For this review, take the finished solid that the model builds, in its own axes (mm). Coordinates: 2 decimals unless noted, no trailing zeros. Order: outer loops, then holes, each group sorted by start corner. A loop starts at its lowest first (then second) coordinate and runs counter-clockwise, first axis right, second up. Notation, with made-up numbers: (28.5, 20.25) -> (57.5, 20.25) arc R31 ccw to (57.5, 47.25) -> close; hole circle Ø11 at (24, -37). An arc over 180 degrees is marked (long way). Answer as a JSON object with one key per item and string values. Group by question number.
1) Draft analysis for pull direction Z (two halves, no side actions). For faces 1 (the flat face through (0, 6, 0)), 2 (the flat face through (0, 3, 2)), 3 (the cylindrical face through (-11.976, 5.423, 6.368)), state which applies: +Z half, -Z half, draft (parallel to the pull), parting line (faces both ways), or undercut.
2) For pin 1 (1.5 mm diameter, centred on x = -3.5, z = 3.5, fed in from -Y), flat-tipped, find the tip position at first contact; note if it passes through.
3) Add section A-A, the plane x = 0. Write out the cut boundary in (y, z), then the cut area to 3 significant figures.
4) Add section D-D, the plane x = -13.5. Write out the cut boundary in (y, z), then the cut area to 3 significant figures.
5) Wall thickness on L1, parallel to Z at x = 13.5, y = 5.75; L2, parallel to Z at x = -15, y = 9.5; L3, parallel to X at y = 8.25, z = 15.75: over which ranges is each line inside the solid? List them lowest first.
6) Add section B-B, the plane y = 9.75. Write out the cut boundary in (x, z), then the cut area to 3 significant figures.
7) Add section C-C, the plane z = 12. Write out the cut boundary in (x, y), then the cut area to 3 significant figures.
from build123d import *

# Parameters (mm, degrees)
EXTRUDE_1_DEPTH     = 22
SKETCH_3_R          = 1.65
CUT_EXTRUDE_2_DEPTH = 19
EXTRUDE_2_DEPTH     = 2
SKETCH_5_R          = 1.65
CUT_EXTRUDE_3_DEPTH = 31.186917806


with BuildPart() as part:
    # 草图1 → 凸台-拉伸1 (new body)
    with BuildSketch(Plane.XY):
        with BuildLine():
            Line((-10.583005244, 3), (-17.5, 3))
            Line((-17.5, 3), (-17.5, 0))
            Line((-17.5, 0), (-11, 0))
            ThreePointArc((-11, 0), (-10.895252583, 1.514421063), (-10.583005244, 3))
        make_face()
        with BuildLine():
            Line((-7.416198487, 3), (-10.583005244, 3))
            ThreePointArc((-10.583005244, 3), (-10.895252583, 1.514421063), (-11, 0))
            Line((-11, 0), (-8, 0))
            ThreePointArc((-8, 0), (-7.85269342, 1.5281381), (-7.416198487, 3))
        make_face()
        with BuildLine():
            ThreePointArc((11, 0), (10.895252583, 1.514421063), (10.583005244, 3))
            Line((10.583005244, 3), (7.416198487, 3))
            ThreePointArc((7.416198487, 3), (7.85269342, 1.5281381), (8, 0))
            Line((8, 0), (11, 0))
        make_face()
        with BuildLine():
            ThreePointArc((-4.5e-08, 11), (-6.633249599, 8.774964374), (-10.583005244, 3))
            Line((-10.583005244, 3), (-7.416198487, 3))
            ThreePointArc((-7.416198487, 3), (0, 8), (7.416198487, 3))
            Line((7.416198487, 3), (10.583005244, 3))
            ThreePointArc((10.583005244, 3), (6.633249563, 8.774964401), (-4.5e-08, 11))
        make_face()
        with BuildLine():
            Line((17.5, 3), (10.583005244, 3))
            ThreePointArc((10.583005244, 3), (10.895252583, 1.514421063), (11, 0))
            Line((11, 0), (17.5, 0))
            Line((17.5, 0), (17.5, 3))
        make_face()
        with BuildLine():
            Line((-17.5, 11), (-17.5, 3))
            Line((-17.5, 3), (-10.583005244, 3))
            ThreePointArc((-10.583005244, 3), (-6.633249599, 8.774964374), (-4.5e-08, 11))
            Line((-4.5e-08, 11), (-17.5, 11))
        make_face()
        with BuildLine():
            Line((17.5, 11), (-4.5e-08, 11))
            ThreePointArc((-4.5e-08, 11), (6.633249563, 8.774964401), (10.583005244, 3))
            Line((10.583005244, 3), (17.5, 3))
            Line((17.5, 3), (17.5, 11))
        make_face()
    extrude(amount=EXTRUDE_1_DEPTH)

    # 草图3 → 切除-拉伸2 (cut)
    with BuildSketch(Plane(origin=(0, 0, 0), x_dir=(1, 0, 0), z_dir=(0, 1, 0))):
        with Locations(Location((0, -12, 0), (0, 0, 90))):
            Circle(SKETCH_3_R)
    extrude(amount=CUT_EXTRUDE_2_DEPTH, mode=Mode.SUBTRACT)

    # 草图4 → 凸台-拉伸2 (add)
    with BuildSketch(Plane(origin=(0, 0, 0), x_dir=(-1, 0, 0), z_dir=(0, 0, -1))):
        with BuildLine():
            Line((-11, 0), (11, 0))
            ThreePointArc((11, 0), (0, 11), (-11, 0))
        make_face()
    extrude(amount=-EXTRUDE_2_DEPTH)

    # 草图5 → 切除-拉伸3 (cut, through all)
    with BuildSketch(Plane.XZ):
        with Locations((-13.5, 17)):
            Circle(SKETCH_5_R)
        with Locations((-13.5, 7)):
            Circle(SKETCH_5_R)
        with Locations((13.5, 17)):
            Circle(SKETCH_5_R)
        with Locations((13.5, 7)):
            Circle(SKETCH_5_R)
    extrude(amount=-CUT_EXTRUDE_3_DEPTH, mode=Mode.SUBTRACT)


solid = part.part
Output values:
{
 "1": {"face 1": "-Z half", "face 2": "+Z half", "face 3": "undercut"},
 "2": {"pin 1": "stops at y = 6.78"},
 "3": {"outline": "(0, 0) -> (11, 0) -> (11, 10.35) -> (8, 10.35) -> (8, 2) -> (0, 2) -> close; (8, 13.65) -> (11, 13.65) -> (11, 22) -> (8, 22) -> close", "area": "72.1 mm²"},
 "4": {"outline": "(0, 0) -> (11, 0) -> (11, 5.35) -> (0, 5.35) -> close; (0, 8.65) -> (11, 8.65) -> (11, 15.35) -> (0, 15.35) -> close; (0, 18.65) -> (11, 18.65) -> (11, 22) -> (0, 22) -> close", "area": "169 mm²"},
 "5": {"L1": "z = 0 to 5.35, 8.65 to 15.35, 18.65 to 22", "L2": "z = 0 to 6.31, 7.69 to 16.31, 17.69 to 22", "L3": "x = -17.5 to -14.58, -12.42 to 12.42, 14.58 to 17.5"},
 "6": {"outline": "(-17.5, 0) -> (17.5, 0) -> (17.5, 22) -> (-17.5, 22) -> close; hole circle Ø3.3 at (-13.5, 7); hole circle Ø3.3 at (-13.5, 17); hole circle Ø3.3 at (0, 12); hole circle Ø3.3 at (13.5, 7); hole circle Ø3.3 at (13.5, 17)", "area": "727 mm²"},
 "7": {"outline": "(-17.5, 0) -> (-8, 0) arc R8 cw to (-1.65, 7.83) -> (-1.65, 11) -> (-17.5, 11) -> close; (1.65, 7.83) arc R8 cw to (8, 0) -> (17.5, 0) -> (17.5, 11) -> (1.65, 11) -> close", "area": "274 mm²"}
}
